Autodesk Inventor part; units mm, degrees
ref_plane "YZ Plane" through (0, 0, 0) normal (1, 0, 0) x (0, 1, 0)
ref_plane "XZ Plane" through (0, 0, 0) normal (0, 1, 0) x (-1, 0, 0)
ref_plane "XY Plane" through (0, 0, 0) normal (0, 0, 1) x (1, 0, 0)
sketch "Sketch1" plane through (0, 0, 0) normal (0, 1, 0) x (-1, 0, 0)
  line L0 (0, 0) -> (130, 0)
  line L1 (130, 0) -> (130, -50)
  line L2 (130, -50) -> (0, -50)
  line L3 (0, -50) -> (0, 0)
  dimension "d0" = 130
  dimension "d1" = 50
extrude "Extrusion1" add sketch "Sketch1" along normal blind 1.27
sketch "Sketch2" plane through (0, 1.27, 0) normal (0, 1, 0) x (1, 0, 0)
  line L0 (-130, 0) -> (0, 0)
  line L1 (0, 0) -> (0, 50)
  line L2 (-130, 0) -> (0, 0)
  line L3 (0, 0) -> (0, 1.27)
  line L4 (0, 1.27) -> (-130, 1.27)
  line L5 (-130, 1.27) -> (-130, 0)
  line L6 (-130, 50) -> (-130, 0)
  line L7 (-130, 50) -> (0, 50)
  line L8 (0, 50) -> (0, 48.73)
  line L9 (0, 48.73) -> (-130, 48.73)
  line L10 (-130, 48.73) -> (-130, 50)
  line L11 (0, 1.27) -> (-1.27, 1.27)
  line L12 (-1.27, 1.27) -> (-1.27, 48.73)
  line L13 (-1.27, 48.73) -> (0, 48.73)
  line L14 (0, 48.73) -> (0, 1.27)
  line L15 (-130, 1.27) -> (-128.73, 1.27)
  line L16 (-128.73, 1.27) -> (-128.73, 48.73)
  line L17 (-128.73, 48.73) -> (-130, 48.73)
  line L18 (-130, 48.73) -> (-130, 1.27)
  dimension "d4" = 1.27
  dimension "d5" = 1.27
  dimension "d6" = 1.27
  dimension "d7" = 1.27
extrude "Extrusion2" add sketch "Sketch2" along normal blind 33.72 contours L5 L4 L1 L0 | L6 L9 L16 L4 | L4 L12 L9 L1 | L6 L7 L1 L9
sketch "Sketch3" plane through (0, 0, 0) normal (1, 0, 0) x (0, 0, -1)
  circle A0 centre (39.3882, 4.5) radius 3.175
  line L0 (50, 0) -> (0, 0)
  dimension "d10" = 6.35
  dimension "d17" = 4.5
extrude "Extrusion3" add sketch "Sketch3" along normal blind 15
sketch "Sketch4" plane through (15, 4.5, -39.3882) normal (1, 0, 0) x (0, 0, -1)
  circle A0 centre (0, 0) radius 1.5
  point P0 (-39.3882, -4.5)
  dimension "d14" = 3
extrude "Extrusion4" cut sketch "Sketch4" against normal blind 30
properties part number "CajaDesague"
The model under review builds one solid part; all positions refer to its coordinate system, in mm. A direction names the side the tool comes from. Round coordinates to 2 decimals unless told otherwise and drop trailing zeros. Loops run counter-clockwise (first coordinate to the right, second up) from the corner with the lowest first, then second, coordinate; pieces in that order, holes last. Notation, with made-up numbers: (-34, 4.25) -> (-17, 4.25) arc R33 ccw to (-17, 35.25) -> close; hole circle Ø1 at (26.5, 59.25). An arc over 180 degrees is marked (long way). Answer in a Markdown table with one row per item.
1) Consider section D-D, the plane x = 1.5. Write out the cut boundary in (y, z) (3 decimals), plus the area to 3 significant figures.
Taken from the geometry:
| item | result |
|---|---|
| outline | circle Ø6.35 at (4.5, -39.388); hole circle Ø3 at (4.5, -39.388) |
| area | 24.6 mm² |
2) For pin 1 Ø14 at (x, z) = (-74.5, -17) entering from +Y; pin 2 Ø8 at (y, z) = (11.5, -18.5) entering from +X, all flat-tipped, find the tip position at first contact; note any pin that passes through.
Taken from the geometry:
| item | result |
|---|---|
| pin 1 | stops at y = 1.27 |
| pin 2 | stops at x = 0 |
3) Consider section A-A, the plane y = 12. Write out the cut boundary in (x, z), plus the area to 3 significant figures.
Taken from the geometry:
| item | result |
|---|---|
| outline | (-130, -50) -> (0, -50) -> (0, 0) -> (-130, 0) -> close; hole (-128.73, -48.73) -> (-1.27, -48.73) -> (-1.27, -1.27) -> (-128.73, -1.27) -> close |
| area | 451 mm² |
4) Draft analysis for pull direction X (two halves, no side actions). For faces 1 (the flat face through (-130, 17, -25)), 2 (the flat face through (-1.27, 18, -25)), 3 (the cylindrical face through (7.395, 4.36, -36.216)), state which applies: pulls with the +X half, pulls with the -X half, needs draft (parallel to the pull), parting line crosses it, or undercut.
Taken from the geometry:
| item | result |
|---|---|
| face 1 | pulls with the -X half |
| face 2 | undercut |
| face 3 | needs draft |
5) Consider section B-B, the plane x = -114. Write out the cut boundary in (y, z).
Taken from the geometry:
| item | result |
|---|---|
| outline | (0, -50) -> (34.99, -50) -> (34.99, -48.73) -> (1.27, -48.73) -> (1.27, -1.27) -> (34.99, -1.27) -> (34.99, 0) -> (0, 0) -> close |
6) Wall thickness on line 1 along X through (y, z) = (27, -36.5); line 2 along Z through (x, y) = (-99.5, 2); line 3 along Y through (x, z) = (-121, -26): over which ranges is each line inside the solid? List them lowest first.
Taken from the geometry:
| item | result |
|---|---|
| line 1 | x = -130 to -128.73, -1.27 to 0 |
| line 2 | z = -50 to -48.73, -1.27 to 0 |
| line 3 | y = 0 to 1.27 |
7) Tool access review of faces 4 (the flat face through (-66, 17, -50)), 5 (the flat face through (-128.73, 18, -25)), 6 (the cylindrical face through (6.98, 4.57, -37.89)): name each direction out of +Z, -Z, +X, -X, +Y, -Y from which nothing blocks a thin tool from reaching the whole face with its end or side.
Taken from the geometry:
| item | result |
|---|---|
| face 4 | -Z, +X, -X, +Y, -Y |
| face 5 | +Y |
| face 6 | +X |
8) Consider section C-C, the plane z = -20. Write out the cut boundary in (x, y), plus the area to 3 significant figures.
Taken from the geometry:
| item | result |
|---|---|
| outline | (-130, 0) -> (0, 0) -> (0, 34.99) -> (-1.27, 34.99) -> (-1.27, 1.27) -> (-128.73, 1.27) -> (-128.73, 34.99) -> (-130, 34.99) -> close |
| area | 251 mm² |
